Could you check a few things on this drawing? It's one solid part, dimensions in mm from its lowest x, y, z. A direction names the side the tool comes from. Round coordinates to 2 decimals unless told otherwise and drop trailing zeros. Write each loop counter-clockwise with the first axis right and the second up, starting at its lowest first coordinate (ties: lowest second). Pieces come first, ordered by that corner, then holes. Notation, with made-up numbers: (22.25, 44.25) - (66.25, 44.25) arc R14 ccw to (66.25, 61.25) - close; hole circle Ø7 at (43.5, 79). An arc over 180 degrees is marked (long way). One line per question, with ' | ' between items. Start each with the question number.
(1) Imagine slicing it at D-D (y = 353). Write out the boundary of the cut face in (x, z), plus the area to 3 significant figures.
(2) If I drill on L1, parallel to Y at x = 244, z = 11.5; L2, parallel to X at y = 224.5, z = 4; L3, parallel to X at y = 149.5, z = 25, over which ranges is the centre line in solid material (lowest first)?
(3) For the marked faces 4 and 5, which set-ups out of +Z, -Z, +X, -X, +Y, -Y let a thin tool reach every point of the face, with its end or its side?
(4) Imagine slicing it at B-B (x = 145). Write out the boundary of the cut face in (y, z).
(5) Imagine slicing it at C-C (z = 50). Write out the boundary of the cut face in (x, y), plus the area to 3 significant figures.
(6) Imagine slicing it at A-A (y = 252). Write out the boundary of the cut face in (x, z), plus the area to 3 significant figures.
(7) Will this pin go through, and if not, where does the flat tip stop? pin 1 (3 mm diameter, centred on x = 133.5, z = 4.5, fed in from -Y).
(8) Thinking about a two-plate mould opening in Y: for the marked faces 1, 2 and 3, which applies, pulls with the +Y half, pulls with the -Y half, needs draft (parallel to the pull), parting line crosses it, or undercut?
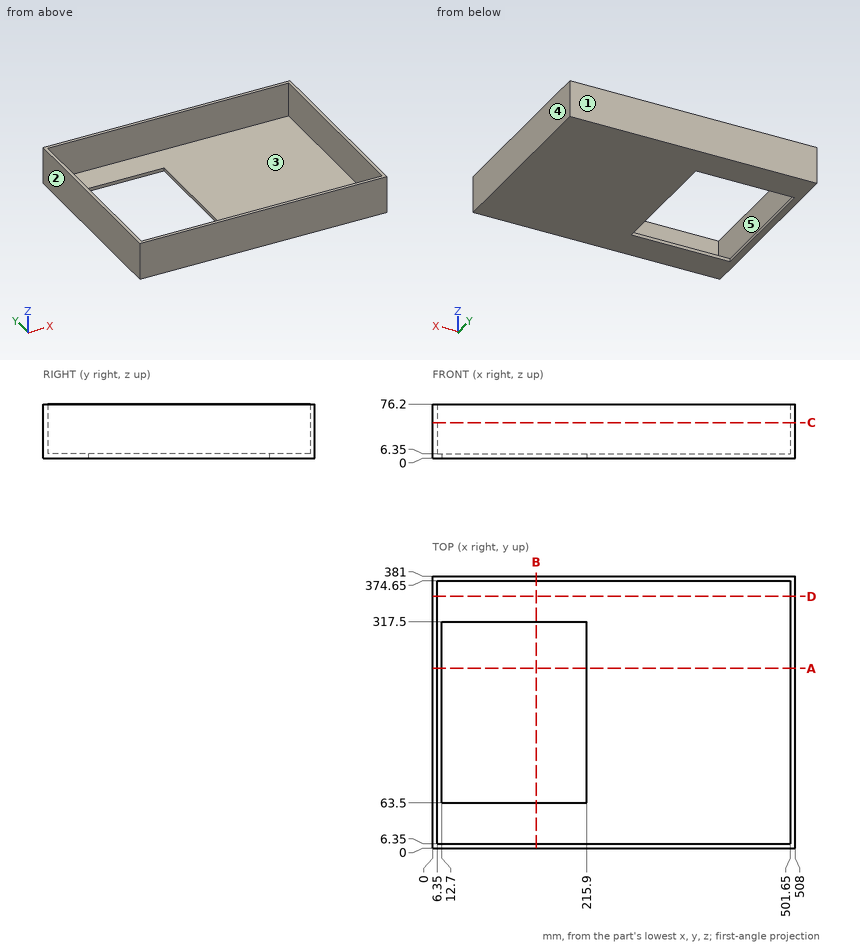
Check sheet entries:
1) outline: (0, 0) - (508, 0) - (508, 76.2) - (501.65, 76.2) - (501.65, 6.35) - (6.35, 6.35) - (6.35, 76.2) - (0, 76.2) - close | area: 4,110 mm^2
2) L1: 0 to 6.35, 374.65 to 381 | L2: 0 to 12.7, 215.9 to 508 | L3: 0 to 6.35, 501.65 to 508
3) face 4: +Z, -Z, +X, +Y, -Y | face 5: +Z
4) outline: (0, 0) - (63.5, 0) - (63.5, 6.35) - (6.35, 6.35) - (6.35, 76.2) - (0, 76.2) - close; (317.5, 0) - (381, 0) - (381, 76.2) - (374.65, 76.2) - (374.65, 6.35) - (317.5, 6.35) - close
5) outline: (0, 0) - (508, 0) - (508, 381) - (0, 381) - close; hole (6.35, 6.35) - (501.65, 6.35) - (501.65, 374.65) - (6.35, 374.65) - close | area: 11,100 mm^2
6) outline: (0, 0) - (12.7, 0) - (12.7, 6.35) - (6.35, 6.35) - (6.35, 76.2) - (0, 76.2) - close; (215.9, 0) - (508, 0) - (508, 76.2) - (501.65, 76.2) - (501.65, 6.35) - (215.9, 6.35) - close | area: 2,820 mm^2
7) pin 1: y = 0
8) face 1: pulls with the +Y half | face 2: needs draft | face 3: undercut
